from build123d import *

# Parameters (mm, degrees)
SKETCH1_R           = 5
BOSS_EXTRUDE1_DEPTH = 2
BOSS_EXTRUDE2_DEPTH = 10
LPATTERN1_COUNT     = 2
LPATTERN1_PITCH     = 12
FILLET1_R           = 1.5
SKETCH3_W           = 56.126339002
SKETCH3_H           = 22.59818153
BOSS_EXTRUDE3_DEPTH = 11
CUT_EXTRUDE1_DEPTH  = 47.406488284
SHELL1_START        = -14.299090765
SHELL1_DEPTH        = 18.59818153
FILLET2_R           = 1.5
SKETCH6_W           = 1.5
SKETCH6_H           = 18.59818153
BOSS_EXTRUDE4_DEPTH = 2


# Read off the part's stored shape, not the designer's step: Shell1
with BuildPart() as part:
    # Sketch1 → Boss-Extrude1 (new body)
    with BuildSketch(Plane.XY):
        with BuildLine():
            Line((-11.361776574, -18.246245298), (-8.801388784, 1.161153468))
            ThreePointArc((-8.801388784, 1.161153468), (0, 8.87765295), (8.801388784, 1.161153468))
            Line((8.801388784, 1.161153468), (11.361776574, -18.246245298))
            Line((11.361776574, -18.246245298), (-11.361776574, -18.246245298))
        make_face()
        Circle(SKETCH1_R, mode=Mode.SUBTRACT)
    boss_extrude1 = extrude(amount=BOSS_EXTRUDE1_DEPTH)

    # Sketch2 → Boss-Extrude2 (add)
    with BuildSketch(Plane(origin=(0, 0, 0), x_dir=(-1, 0, 0), z_dir=(0, 0, -1))):
        Polygon((-11.0979197, -16.246245298), (11.0979197, -16.246245298), (11.361776574, -18.246245298), (-11.361776574, -18.246245298), align=None)
    extrude(amount=BOSS_EXTRUDE2_DEPTH)

    # LPattern1: Boss-Extrude1 ×2
    with Locations(*[(0, 0, -i * LPATTERN1_PITCH) for i in range(1, LPATTERN1_COUNT)]):
        add(boss_extrude1)

    # Fillet1
    fillet1_edges = [part.edges().sort_by_distance(p)[0] for p in [
        (0, -18.246245298, -12),
        (0, -16.246245298, 0),
        (0, -16.246245298, -10),
        (0, -18.246245298, 2),
    ]]
    fillet(fillet1_edges, radius=FILLET1_R)

    # Sketch3 → Boss-Extrude3 (add)
    with BuildSketch(Plane.XZ.offset(18.246245298)):
        with Locations((0, -5)):
            Rectangle(SKETCH3_W, SKETCH3_H)
    extrude(amount=BOSS_EXTRUDE3_DEPTH)

    # Sketch5 → Cut-Extrude1 (cut, through all)
    with BuildSketch(Plane.XY.offset(6.299090765)):
        Polygon((-28.063169501, -29.246245298), (-24.755567795, -18.246245298), (-28.063169501, -18.246245298), align=None)
        Polygon((28.063169501, -18.246245298), (28.063169501, -29.246245298), (24.755567795, -18.246245298), align=None)
    extrude(amount=-CUT_EXTRUDE1_DEPTH, mode=Mode.SUBTRACT)

    # Shell1 outline → Shell1 (cut)
    with BuildSketch(Plane.XY.offset(SHELL1_START)):
        Polygon((25.974710628, -29.246245298), (25.674019564, -28.246245298), (-25.674019564, -28.246245298), (-25.974710628, -29.246245298), align=None)
    extrude(amount=SHELL1_DEPTH, mode=Mode.SUBTRACT)

    # Fillet2
    fillet2_edges = [part.edges().sort_by_distance(p)[0] for p in [
        (26.409368648, -23.746245298, -16.299090765),
        (26.409368648, -23.746245298, 6.299090765),
        (25.824365096, -28.746245298, -14.299090765),
        (-25.824365096, -28.746245298, -14.299090765),
        (-25.824365096, -28.746245298, 4.299090765),
        (25.824365096, -28.746245298, 4.299090765),
        (-26.409368648, -23.746245298, -16.299090765),
        (-26.409368648, -23.746245298, 6.299090765),
    ]]
    fillet(fillet2_edges, radius=FILLET2_R)

    # Sketch6 → Boss-Extrude4 (add)
    with BuildSketch(Plane.XZ.offset(28.246245298)):
        with Locations((23.658366473, -5)):
            Rectangle(SKETCH6_W, SKETCH6_H)
        with Locations((20.038366473, -5)):
            Rectangle(SKETCH6_W, SKETCH6_H)
        with Locations((16.418366473, -5)):
            Rectangle(SKETCH6_W, SKETCH6_H)
        with Locations((12.798366473, -5)):
            Rectangle(SKETCH6_W, SKETCH6_H)
        with Locations((9.178366473, -5)):
            Rectangle(SKETCH6_W, SKETCH6_H)
        with Locations((5.558366473, -5)):
            Rectangle(SKETCH6_W, SKETCH6_H)
        with Locations((1.938366473, -5)):
            Rectangle(SKETCH6_W, SKETCH6_H)
        with Locations((-1.681633527, -5)):
            Rectangle(SKETCH6_W, SKETCH6_H)
        with Locations((-5.301633527, -5)):
            Rectangle(SKETCH6_W, SKETCH6_H)
        with Locations((-8.921633527, -5)):
            Rectangle(SKETCH6_W, SKETCH6_H)
        with Locations((-12.541633527, -5)):
            Rectangle(SKETCH6_W, SKETCH6_H)
        with Locations((-16.161633527, -5)):
            Rectangle(SKETCH6_W, SKETCH6_H)
        with Locations((-19.781633527, -5)):
            Rectangle(SKETCH6_W, SKETCH6_H)
        with Locations((-23.401633527, -5)):
            Rectangle(SKETCH6_W, SKETCH6_H)
    extrude(amount=BOSS_EXTRUDE4_DEPTH)


solid = part.part
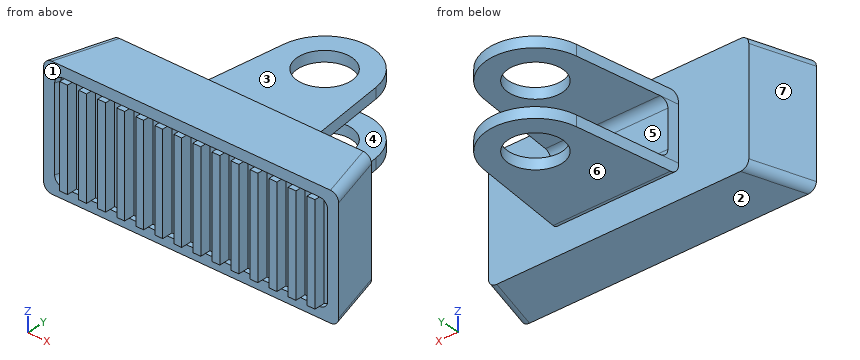
Work out the finished part from the listing and answer in its coordinate system (mm). Face numbers are marked on the shaded views. A direction names the side the tool comes from. Give positions to 0.01 mm unless a question says otherwise; leave off trailing zeros. Write each loop counter-clockwise with the first axis right and the second up, starting at its lowest first coordinate (ties: lowest second). Pieces come first, ordered by that corner, then holes.
Q1. The part is cut by section C-C on y = -10. Give the vertices of the cut face in (x, z).
Answer:
outline: (-10.27, -12) - (10.27, -12) - (10.27, -10) - (-10.27, -10) - close; (-10.27, 0) - (10.27, 0) - (10.27, 2) - (-10.27, 2) - close
Q2. Straight lines are drawn through the part: L1, parallel to Z at x = 4, y = 5.5; L2, parallel to Y at x = 7, z = 1.75; L3, parallel to Y at x = 16, z = 5. For each, find the intervals that lie inside material, in ascending order.
Answer:
L1: z = -12 to -10, 0 to 2
L2: y = -28.25 to -18.25, -17.58 to 5.46
L3: y = -29.25 to -18.25
Q3. The part is cut by section B-B on y = 0. Give the vertices of the cut face in (x, z), and give its area (3 significant figures).
Answer:
outline: (-8.95, -12) - (-5, -12) - (-5, -10) - (-8.95, -10) - close; (-8.95, 0) - (-5, 0) - (-5, 2) - (-8.95, 2) - close; (5, -12) - (8.95, -12) - (8.95, -10) - (5, -10) - close; (5, 0) - (8.95, 0) - (8.95, 2) - (5, 2) - close
area: 31.6 mm2
Q4. Given pin 1 (1.1 mm diameter, centred on x = 0, z = -4, fed in from -Y); pin 2 (1 mm diameter, centred on x = -11.5, z = -1.5, fed in from +Y); pin 3 (5 mm diameter, centred on y = 4, z = -8, fed in from -X), each flat-ended and moving along its own axis, determine where each tip first touches the part or whether it passes through.
Answer:
pin 1: stops at y = -28.25
pin 2: stops at y = -16.22
pin 3: stops at x = -8.52
Q5. For a pull along Z with two mould halves and no side action, classify the marked faces 1, 2, 3 and 4 as released by +Z, released by -Z, zero draft, split by the parting line, or undercut.
Answer:
face 1: zero draft
face 2: released by -Z
face 3: released by +Z
face 4: undercut
Q6. A tool of negligible diameter and unlimited length cuts with its end or side. For the marked faces 5, 6 and 7, from which of +Z, -Z, +X, -X, +Y, -Y can it reach the whole face along a straight path? Write none if from no direction.
Answer:
face 5: +X, -X, +Y
face 6: -Z, +X, -X, +Y
face 7: +Z, -Z, -X, +Y
Q7. The part is cut by section A-A on x = 0. Give the vertices of the cut face in (y, z), and give its area (3 significant figures).
Answer:
outline: (-29.25, -16.3) - (-18.25, -16.3) - (-18.25, -10.5) arc R1.5 ccw to (-16.75, -12) - (-5, -12) - (-5, -10) - (-14.75, -10) arc R1.5 cw to (-16.25, -8.5) - (-16.25, -1.5) arc R1.5 cw to (-14.75, 0) - (-5, 0) - (-5, 2) - (-16.75, 2) arc R1.5 ccw to (-18.25, 0.5) - (-18.25, 6.3) - (-29.25, 6.3) - (-29.25, 4.3) - (-28.25, 4.3) - (-28.25, -14.3) - (-29.25, -14.3) - close; (5, -12) - (8.88, -12) - (8.88, -10) - (5, -10) - close; (5, 0) - (8.88, 0) - (8.88, 2) - (5, 2) - close
area: 318 mm2
